Can you work these out from the model? Positions are in its coordinate system, mm. Round coordinates to 2 decimals unless told otherwise and drop trailing zeros. Loops run counter-clockwise (first coordinate to the right, second up) from the corner with the lowest first, then second, coordinate; pieces in that order, holes last. Notation, with made-up numbers: (61, 12) -> (105, 12) arc R27 ccw to (105, 50) -> close; hole circle Ø2 at (15, 0). An arc over 180 degrees is marked (long way). Use a Markdown table: item, result.
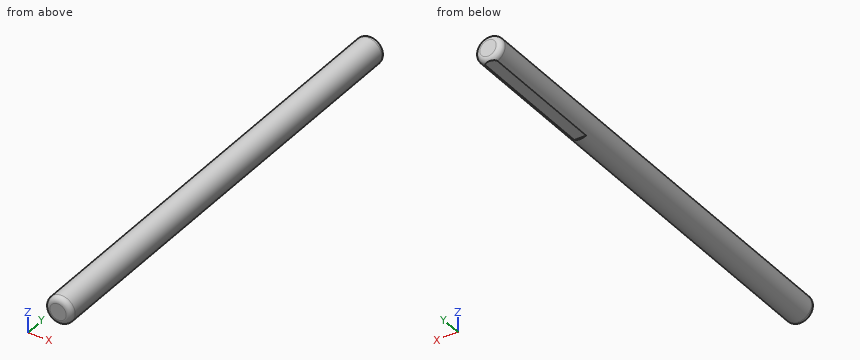
from build123d import *

# Parameters (mm, degrees)
SKETCH2_R           = 2.5
BOSS_EXTRUDE1_DEPTH = 85
CUT_EXTRUDE1_START  = -25
CUT_EXTRUDE1_DEPTH  = 25
FILLET1_R           = 1
FILLET2_R           = 1


with BuildPart() as part:
    # Sketch2 → Boss-Extrude1 (new body)
    with BuildSketch(Plane(origin=(0, 0, 0), x_dir=(1, 0, 0), z_dir=(0, 1, 0))):
        with Locations(Location((0.061061942, 0.061061942, 0), (0, 0, 270))):
            Circle(SKETCH2_R)
    extrude(amount=BOSS_EXTRUDE1_DEPTH)

    # Sketch3 → Cut-Extrude1 (cut)
    with BuildSketch(Plane(origin=(0, 85, 0), x_dir=(1, 0, 0), z_dir=(0, 1, 0)).offset(CUT_EXTRUDE1_START)):
        with BuildLine():
            Line((-1.00625914, 2.321775482), (1.173082806, 2.300126389))
            ThreePointArc((1.173082806, 2.300126389), (0.085895154, 2.560938601), (-1.00625914, 2.321775482))
        make_face()
    extrude(amount=CUT_EXTRUDE1_DEPTH, mode=Mode.SUBTRACT)

    # Fillet1
    # the kernel refuses this fillet: 1 mm, written as the material it takes off along each edge
    with BuildSketch(Plane(origin=(0.061061942, 85, -0.061061942), x_dir=(0.5312663336495629, 0, -0.8472048646759243), z_dir=(0.8472048646759243, 0, 0.5312663336495629))) as fillet1_piece_1:
        with BuildLine():
            CenterArc((2.5 - FILLET1_R, -FILLET1_R), FILLET1_R, 0, 90)
            Line((2.5 - FILLET1_R, 0), (2.5, 0))
            Line((2.5, 0), (2.5, -FILLET1_R))
        make_face()
    revolve(axis=Axis((0.061061942, 85, -0.061061942), (0, 1, 0)), revolution_arc=212.091055881, mode=Mode.SUBTRACT)
    with BuildSketch(Plane(origin=(0.061061942, 85, -0.061061942), x_dir=(0, 0, 1), z_dir=(-1, 0, 0))) as fillet1_piece_2:
        with BuildLine():
            CenterArc((2.5 - FILLET1_R, -FILLET1_R), FILLET1_R, 0, 90)
            Line((2.5 - FILLET1_R, 0), (2.5, 0))
            Line((2.5, 0), (2.5, -FILLET1_R))
        make_face()
    revolve(axis=Axis((0.061061942, 85, -0.061061942), (0, 1, 0)), revolution_arc=210.951767977, mode=Mode.SUBTRACT)

    # Fillet2
    fillet2_edges = [part.edges().sort_by_distance(p)[0] for p in [
        (0.061061942, 0, -2.561061942),
    ]]
    fillet(fillet2_edges, radius=FILLET2_R)


solid = part.part
1. I want a section at A-A (y = 73). Please give me the cut outline in (x, z), plus the area to 3 significant figures.
Answer sheet:
| item | result |
|---|---|
| outline | (-1.01, -2.32) -> (1.17, -2.3) arc R2.5 ccw (long way) to start |
| area | 19.3 mm² |
2. I want a section at B-B (y = 20). Please give me the cut outline in (x, z), plus the area to 3 significant figures.
Answer sheet:
| item | result |
|---|---|
| outline | circle Ø5 at (0.06, -0.06) |
| area | 19.6 mm² |
3. I need wall thicknesses on line 1 (Z direction, x = 0.1, y = 70.5); line 2 (Y direction, x = 1.65, z = 0.1); line 3 (Z direction, x = -0.15, y = 19). Which ranges of each line are inside material? Lowest first, please.
Answer sheet:
| item | result |
|---|---|
| line 1 | z = -2.31 to 2.44 |
| line 2 | y = 0 to 85 |
| line 3 | z = -2.55 to 2.43 |
